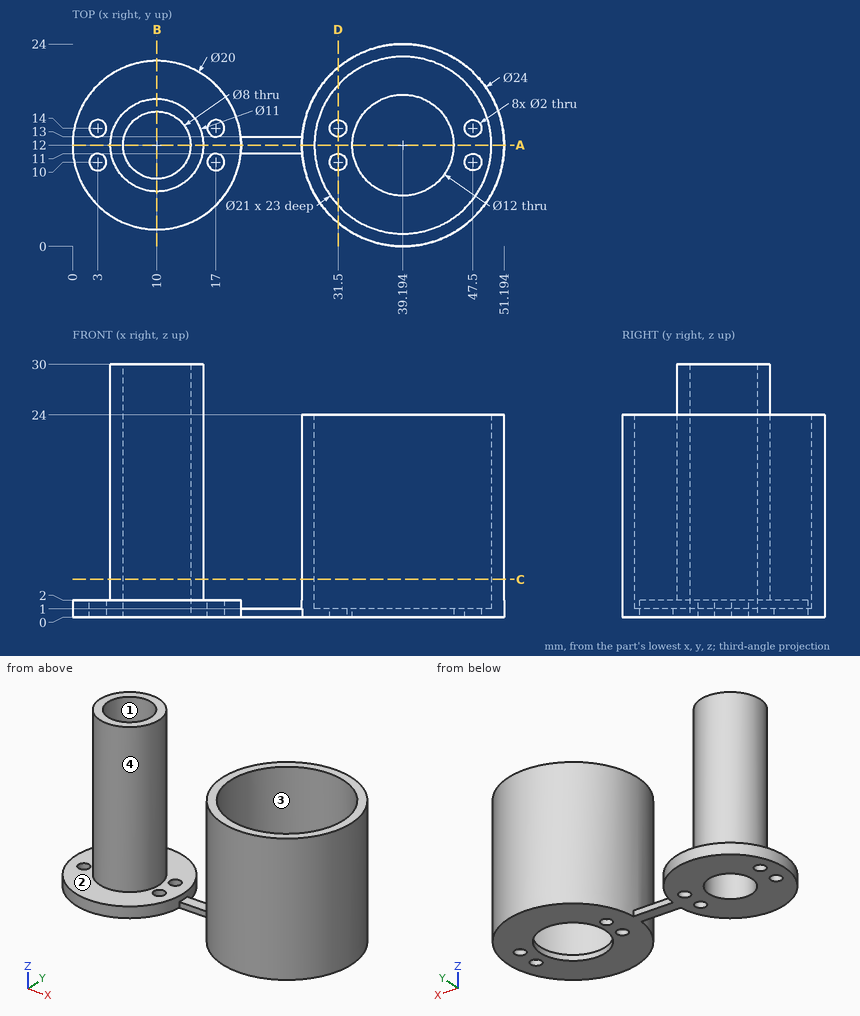
The figure shows three views and two pictorial views of one solid part (mm, origin at its lowest corner). Answer the questions. Coordinates: 2 decimals unless noted, no trailing zeros. Loops run counter-clockwise (first coordinate to the right, second up) from the corner with the lowest first, then second, coordinate; pieces in that order, holes last. Notation, with made-up numbers: (-22.75, -14) -> (33.25, -14) arc R16 cw to (33.25, -9) -> close; hole circle Ø1 at (56.5, -16.75). An arc over 180 degrees is marked (long way). Return JSON: item names as keys, results as strings. Group by question number.
(1) Given pin 1 Ø12 at (y, z) = (5, 21.5) entering from +X; pin 2 Ø12 at (x, y) = (42, 14.5) entering from +Z; pin 3 Ø1.1 at (x, z) = (24.5, 0.5) entering from -Y; pin 4 Ø1.8 at (x, y) = (47.5, 10) entering from +Z, each flat-ended and moving along its own axis, determine where each tip first touches the part or whether it passes through.
(2) A cutting plane is placed at C-C on z = 4.5. Write down the section's boundary in (x, y).
(3) Find the intervals of material crossed by probe 1 along X at (y, z) = (14.5, 18.5) (1 decimal); probe 2 along Y at (x, z) = (31.5, 0.5); probe 3 along X at (y, z) = (15, 23.5) (1 decimal), in increasing order. Write a range as from..to.
(4) A cutting plane is placed at A-A on y = 12. Write down the section's boundary in (x, z).
(5) A cutting plane is placed at B-B on x = 10. Write down the section's boundary in (y, z).
(6) A cutting plane is placed at D-D on x = 31.5. Write down the section's boundary in (y, z) (1 decimal).
(7) Determine the mould class of the marked faces 1, 2, 3 and 4 for opening direction Y: released by +Y, released by -Y, zero draft, split by the parting line, or undercut.
The answers:
{
 "1": {"pin 1": "stops at x = 51.15", "pin 2": "stops at z = 1", "pin 3": "stops at y = 11", "pin 4": "passes through"},
 "2": {"outline": "circle Ø11 at (10, 12); circle Ø24 at (39.19, 12); hole circle Ø8 at (10, 12); hole circle Ø21 at (39.19, 12)"},
 "3": {"probe 1": "x = 5.1..6.9, 13.1..14.9, 27.5..29, 49.4..50.9", "probe 2": "y = 2.79..9, 11..13, 15..21.21", "probe 3": "x = 5.4..7.4, 12.6..14.6, 27.6..29.1, 49.3..50.8"},
 "4": {"outline": "(0, 0) -> (6, 0) -> (6, 30) -> (4.5, 30) -> (4.5, 2) -> (0, 2) -> close; (14, 0) -> (33.19, 0) -> (33.19, 1) -> (28.69, 1) -> (28.69, 24) -> (27.19, 24) -> (27.19, 1) -> (20, 1) -> (20, 2) -> (15.5, 2) -> (15.5, 30) -> (14, 30) -> close; (45.19, 0) -> (51.19, 0) -> (51.19, 24) -> (49.69, 24) -> (49.69, 1) -> (45.19, 1) -> close"},
 "5": {"outline": "(2, 0) -> (8, 0) -> (8, 30) -> (6.5, 30) -> (6.5, 2) -> (2, 2) -> close; (16, 0) -> (22, 0) -> (22, 2) -> (17.5, 2) -> (17.5, 30) -> (16, 30) -> close"},
 "6": {"outline": "(2.8, 0) -> (9, 0) -> (9, 1) -> (4.9, 1) -> (4.9, 24) -> (2.8, 24) -> close; (11, 0) -> (13, 0) -> (13, 1) -> (11, 1) -> close; (15, 0) -> (21.2, 0) -> (21.2, 24) -> (19.1, 24) -> (19.1, 1) -> (15, 1) -> close"},
 "7": {"face 1": "undercut", "face 2": "zero draft", "face 3": "undercut", "face 4": "split by the parting line"}
}
